Input: dimensioned drawing with shaded views. Units: mm. Origin: part minimum x, y, z. Give positions to 0.01 mm unless a question says otherwise; leave off trailing zeros. Loops run counter-clockwise (first coordinate to the right, second up) from the corner with the lowest first, then second, coordinate; pieces in that order, holes last. Notation, with made-up numbers: M -37.75,-30.5 L -4.75,-30.5 A23 ccw -4.75,-17.5 Z; hole C -27.75,85 d11. An arc over 180 degrees is marked long. Answer in a Markdown table with one row per item.
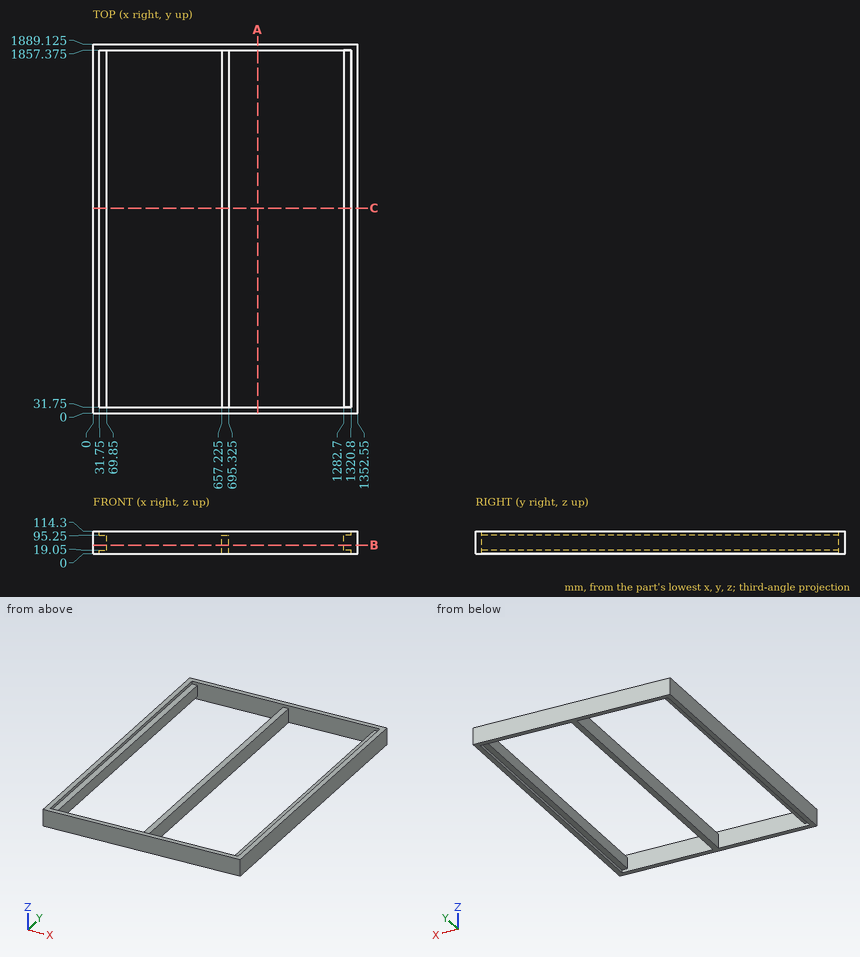
Q1. Ray query, probe 1 along X at (y, z) = (1066.5, 58) (3 decimals); probe 2 along Y at (x, z) = (195.5, 107) (3 decimals); probe 3 along X at (y, z) = (1136, 97.5). Return the intervals inside material, ascending. Write a range as from..to.
Values follow:
| item | result |
|---|---|
| probe 1 | 0..69.85, 657.225..695.325, 1282.7..1352.55 |
| probe 2 | 0..31.75, 1857.375..1889.125 |
| probe 3 | 0..31.75, 1320.8..1352.55 |
Q2. Section query C-C (y = 1049.5). Output: boundary loops of the cut face in (x, z) (3 decimals), plus the area to 3 significant figures.
Values follow:
| item | result |
|---|---|
| outline | M 0,0 L 31.75,0 L 31.75,19.05 L 69.85,19.05 L 69.85,95.25 L 31.75,95.25 L 31.75,114.3 L 0,114.3 Z; M 657.225,0 L 695.325,0 L 695.325,95.25 L 657.225,95.25 Z; M 1282.7,19.05 L 1320.8,19.05 L 1320.8,0 L 1352.55,0 L 1352.55,114.3 L 1320.8,114.3 L 1320.8,95.25 L 1282.7,95.25 Z |
| area | 16,700 mm^2 |
Q3. Section query A-A (x = 842). Output: boundary loops of the cut face in (y, z) (3 decimals), plus the area to 3 significant figures.
Values follow:
| item | result |
|---|---|
| outline | M 0,0 L 31.75,0 L 31.75,114.3 L 0,114.3 Z; M 1857.375,0 L 1889.125,0 L 1889.125,114.3 L 1857.375,114.3 Z |
| area | 7,260 mm^2 |
Q4. Section query B-B (z = 44). Output: boundary loops of the cut face in (x, y) (3 decimals).
Values follow:
| item | result |
|---|---|
| outline | M 0,0 L 1352.55,0 L 1352.55,1889.125 L 0,1889.125 Z; hole M 69.85,31.75 L 657.225,31.75 L 657.225,1857.375 L 69.85,1857.375 Z; hole M 695.325,31.75 L 1282.7,31.75 L 1282.7,1857.375 L 695.325,1857.375 Z |
Q5. Contact query for flat-ended pins moving along their axis: pin 1 Ø5 at (x, y) = (687.5, 484.5) entering from +Z; pin 2 Ø19 at (x, y) = (1310, 795) entering from -Z; pin 3 Ø9.5 at (y, z) = (1281, 9) entering from -X. Output: stop coordinate, or through.
Values follow:
| item | result |
|---|---|
| pin 1 | z = 95.25 |
| pin 2 | z = 19.05 |
| pin 3 | x = 0 |
